Verification items for this drawing (mm, ordinates from the low corner). A direction names the side the tool comes from. Give positions to 0.01 mm unless a question says otherwise; leave off trailing zeros. Loops run counter-clockwise (first coordinate to the right, second up) from the corner with the lowest first, then second, coordinate; pieces in that order, holes last. Notation, with made-up numbers: M -3.5,75.5 L 50.5,75.5 A18 cw 50.5,98.5 Z; hole C -34,87 d11. An arc over 180 degrees is marked long. Use one line per item in the form item = value.
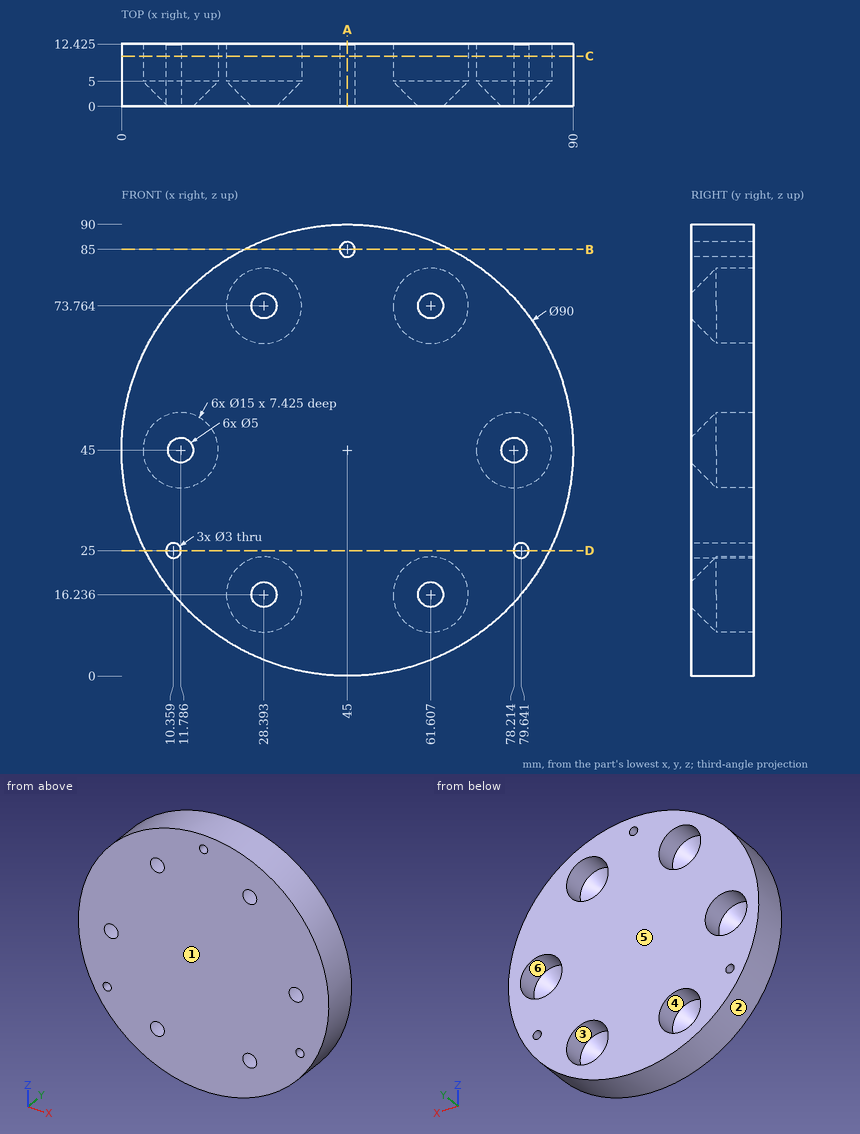
1) Section check B-B (z = 85). Record the cut outline in (x, y) (1 decimal).
Evaluation:
outline = M 24.4,0 L 43.5,0 L 43.5,12.4 L 24.4,12.4 Z; M 46.5,0 L 65.6,0 L 65.6,12.4 L 46.5,12.4 Z
2) Set-up check for the marked faces 5 and 6: record each of +Z, -Z, +X, -X, +Y, -Y from which the full face is reachable in a straight line by a thin tool's end or side.
Evaluation:
face_5 = +Z, -Z, +X, -X, +Y
face_6 = +Y
3) Section check A-A (x = 45). Record the cut outline in (y, z) (1 decimal), then the cut area to 3 significant figures.
Evaluation:
outline = M 0,0 L 12.4,0 L 12.4,83.5 L 0,83.5 Z; M 0,86.5 L 12.4,86.5 L 12.4,90 L 0,90 Z
area = 1,080 mm^2
4) Section check C-C (y = 10). State how many separate pieces and enclosed holes the cut face has, then the cut area to 3 significant figures.
Evaluation:
separate_pieces = 1
enclosed_holes = 9
area = 5,280 mm^2
5) Section check D-D (z = 25). Record the cut outline in (x, y) (1 decimal).
Evaluation:
outline = M 4.7,0 L 8.9,0 L 8.9,12.4 L 4.7,12.4 Z; M 11.9,0 L 78.1,0 L 78.1,12.4 L 11.9,12.4 Z; M 81.1,0 L 85.3,0 L 85.3,12.4 L 81.1,12.4 Z
6) Scan lines: line 1 (X direction, y = 9.25, z = 45); line 2 (Z direction, x = 29, y = 10.5); line 3 (Z direction, x = 28, y = 1.5) (1 decimal). Record each from-to range of solid material in increasing order.
Evaluation:
line_1 = 0 to 4.29, 19.29 to 70.71, 85.71 to 90
line_2 = 2.94 to 8.76, 23.71 to 66.29, 81.24 to 87.06
line_3 = 3.3 to 12.3, 20.2 to 69.8, 77.7 to 86.7
7) Release check for a two-part mould opening along Z. For the marked faces 1, 2, 3 and 4 record: pulls with the +Z half, pulls with the -Z half, needs draft (parallel to the pull), parting line crosses it, or undercut.
Evaluation:
face_1 = needs draft
face_2 = parting line crosses it
face_3 = undercut
face_4 = undercut
8) Depth check by flat-ended pin: pin 1 Ø1.5 at (y, z) = (7, 37) entering from +X; pin 2 Ø5 at (y, z) = (2, 38.5) entering from +X; pin 3 Ø1.5 at (y, z) = (3.5, 42) entering from +X; pin 4 Ø2.5 at (x, z) = (45, 85) entering from +Y. Enter the tip coordinate at first touch or a pass-through.
Evaluation:
pin_1 = 89.41
pin_2 = 89.82
pin_3 = 89.94
pin_4 = through
